```python
from build123d import *

# Parameters (mm, degrees)
SKETCH_1_W           = 55
SKETCH_1_H           = 53
EXTRUDE_1_DEPTH      = 16
SKETCH_3_R           = 2.65
CUT_EXTRUDE_2_DEPTH  = 79.038452061
SKETCH_4_W           = 9.5
SKETCH_4_H           = 12.75
CUT_EXTRUDE_3_DEPTH  = 79.038452061
SKETCH_2_W           = 12
SKETCH_2_H           = 53
CUT_EXTRUDE_4_DEPTH  = 4
SKETCH_5_W           = 12
SKETCH_5_H           = 46
CUT_EXTRUDE_5_DEPTH  = 9
FILLET_1_R           = 2
CUT_EXTRUDE_6_DEPTH  = 79.038452061
FILLET_2_R           = 2
SKETCH_12_W          = 55.94515333
SKETCH_12_H          = 33.208956196
CUT_EXTRUDE_10_DEPTH = 6
SKETCH_13_R          = 1.15
CUT_EXTRUDE_11_DEPTH = 70.756720106
SKETCH_11_W          = 3
SKETCH_11_H          = 46
CUT_EXTRUDE_9_DEPTH  = 13
CUT_EXTRUDE_12_DEPTH = 1
SKETCH_15_R          = 3
SKETCH_15_R_2        = 2.95
CUT_EXTRUDE_13_DEPTH = 12.75
SKETCH_16_R          = 4
CUT_EXTRUDE_14_DEPTH = 2


with BuildPart() as part:
    # 草图1 → 凸台-拉伸1 (new body)
    with BuildSketch(Plane.XY):
        with Locations((-27.5, 26.5)):
            Rectangle(SKETCH_1_W, SKETCH_1_H)
    extrude(amount=EXTRUDE_1_DEPTH)

    # 草图3 → 切除-拉伸2 (cut, through all)
    with BuildSketch(Plane.XZ):
        with Locations(Location((-43, 8, 0), (0, 0, 270))):
            Circle(SKETCH_3_R)
        with Locations(Location((-7, 8, 0), (0, 0, 270))):
            Circle(SKETCH_3_R)
    extrude(amount=-CUT_EXTRUDE_2_DEPTH, mode=Mode.SUBTRACT)

    # 草图4 → 切除-拉伸3 (cut, through all)
    with BuildSketch(Plane.XZ):
        with Locations((-25, 6.375)):
            Rectangle(SKETCH_4_W, SKETCH_4_H)
    extrude(amount=-CUT_EXTRUDE_3_DEPTH, mode=Mode.SUBTRACT)

    # 草图2 → 切除-拉伸4 (cut)
    with BuildSketch(Plane.XY.offset(16)):
        with Locations((-43, 26.5)):
            Rectangle(SKETCH_2_W, SKETCH_2_H)
        with Locations((-6, 26.5)):
            Rectangle(SKETCH_2_W, SKETCH_2_H)
    extrude(amount=-CUT_EXTRUDE_4_DEPTH, mode=Mode.SUBTRACT)

    # 草图5 → 切除-拉伸5 (cut)
    with BuildSketch(Plane.XY.offset(12)):
        with Locations((-43, 30)):
            Rectangle(SKETCH_5_W, SKETCH_5_H)
        with Locations((-6, 30)):
            Rectangle(SKETCH_5_W, SKETCH_5_H)
    extrude(amount=-CUT_EXTRUDE_5_DEPTH, mode=Mode.SUBTRACT)

    # 圆角1
    fillet_1_edges = [part.edges().sort_by_distance(p)[0] for p in [
        (0, 0, 6),
        (0, 53, 1.5),
        (-55, 53, 8),
        (-55, 0, 8),
    ]]
    fillet(fillet_1_edges, radius=FILLET_1_R)

    # 草图6 → 切除-拉伸6 (cut, through all)
    with BuildSketch(Plane.XY.offset(16)):
        with BuildLine():
            Line((-49, 0), (-49, 53))
            Line((-49, 53), (-53, 53))
            ThreePointArc((-53, 53), (-54.414213562, 52.414213562), (-55, 51))
            Line((-55, 51), (-55, 2))
            ThreePointArc((-55, 2), (-54.414213562, 0.585786438), (-53, 0))
            Line((-53, 0), (-49, 0))
        make_face()
    extrude(amount=-CUT_EXTRUDE_6_DEPTH, mode=Mode.SUBTRACT)

    # 圆角2
    fillet_2_edges = [part.edges().sort_by_distance(p)[0] for p in [
        (-49, 53, 1.5),
        (-49, 0, 6),
    ]]
    fillet(fillet_2_edges, radius=FILLET_2_R)

    # 草图12 → 切除-拉伸10 (cut)
    with BuildSketch(Plane(origin=(0, 53, 0), x_dir=(1, 0, 0), z_dir=(0, 1, 0))):
        with Locations((-25.829443508, -5.558164986)):
            Rectangle(SKETCH_12_W, SKETCH_12_H)
    extrude(amount=-CUT_EXTRUDE_10_DEPTH, mode=Mode.SUBTRACT)

    # 草图13 → 切除-拉伸11 (cut, through all)
    with BuildSketch(Plane.XY.offset(16)):
        with Locations((-26.5, 43)):
            Circle(SKETCH_13_R)
        with Locations((-20, 43)):
            Circle(SKETCH_13_R)
    extrude(amount=-CUT_EXTRUDE_11_DEPTH, mode=Mode.SUBTRACT)

    # 草图11 → 切除-拉伸9 (cut)
    with BuildSketch(Plane.XY.offset(16)):
        with Locations((-35.5, 30)):
            Rectangle(SKETCH_11_W, SKETCH_11_H)
        with Locations((-13.5, 30)):
            Rectangle(SKETCH_11_W, SKETCH_11_H)
    extrude(amount=-CUT_EXTRUDE_9_DEPTH, mode=Mode.SUBTRACT)

    # 草图14 → 切除-拉伸12 (cut)
    with BuildSketch(Plane.XY.offset(16)):
        Polygon((-34, 47), (-34, 7), (-37, 7), (-37, 0), (-12, 0), (-12, 7), (-15, 7), (-15, 47), align=None)
    extrude(amount=-CUT_EXTRUDE_12_DEPTH, mode=Mode.SUBTRACT)

    # 草图15 → 切除-拉伸13 (cut)
    with BuildSketch(Plane(origin=(0, 0, 0), x_dir=(-1, 0, 0), z_dir=(0, 0, -1))):
        with Locations((26.5, 43)):
            Circle(SKETCH_15_R)
        with Locations((20, 43)):
            Circle(SKETCH_15_R_2)
    extrude(amount=-CUT_EXTRUDE_13_DEPTH, mode=Mode.SUBTRACT)

    # 草图16 → 切除-拉伸14 (cut)
    with BuildSketch(Plane(origin=(0, 47, 0), x_dir=(1, 0, 0), z_dir=(0, 1, 0))):
        with Locations((-17, -8)):
            Circle(SKETCH_16_R)
        with Locations((-33, -8)):
            Circle(SKETCH_16_R)
    extrude(amount=-CUT_EXTRUDE_14_DEPTH, mode=Mode.SUBTRACT)


solid = part.part
```
Geometry: final body of the model. Coordinates: model frame, mm. A direction names the side the tool comes from. Coordinates: 2 decimals unless noted, no trailing zeros. Order: outer loops, then holes, each group sorted by start corner. A loop starts at its lowest first (then second) coordinate and runs counter-clockwise, first axis right, second up.
Item 1: Section query D-D (x = -33). Output: boundary loops of the cut face in (y, z).
Answer:
outline: (0, 0) - (47, 0) - (47, 4) - (45, 4) - (45, 12) - (47, 12) - (47, 15) - (0, 15) - close
Item 2: Contact query for flat-ended pins moving along their axis: P1, Ø2.5, axis at y = 4.5, z = 13.5, coming from the +X side; P2, Ø3.5, axis at x = -26.5, y = 43, coming from the -Z side; P3, Ø5.5, axis at x = -42, y = 2.5, coming from the +Z side. Output: stop coordinate, or through.
Answer:
P1: stops at x = -12
P2: stops at z = 12.75
P3: stops at z = 12
Item 3: Section query B-B (x = -7). Output: boundary loops of the cut face in (y, z), then the cut area to 3 significant figures.
Answer:
outline: (0, 0) - (47, 0) - (47, 3) - (7, 3) - (7, 5.35) - (0, 5.35) - close; (0, 10.65) - (7, 10.65) - (7, 12) - (0, 12) - close
area: 167 mm2
Item 4: Section query C-C (z = 8). Output: boundary loops of the cut face in (x, y), then the cut area to 3 significant figures.
Answer:
outline: (-49, 2) arc R2 ccw to (-47, 0) - (-45.65, 0) - (-45.65, 7) - (-49, 7) - close; (-40.35, 0) - (-29.75, 0) - (-29.75, 45) - (-34, 45) - (-34, 7) - (-40.35, 7) - close; (-20.25, 0) - (-9.65, 0) - (-9.65, 7) - (-15, 7) - (-15, 45) - (-17.83, 45) arc R2.95 cw to (-20.25, 40.06) - close; (-4.35, 0) - (-2, 0) arc R2 ccw to (0, 2) - (0, 7) - (-4.35, 7) - close
area: 548 mm2
Item 5: Access query for faces 4 (the face through (-43, 4, 12)), 5 (the face through (-20.25, 46.5, 2.8)), 6 (the face through (-6, 4, 12)), 7 (the face through (-8, 27, 3)), 8 (the face through (-17, 46, 12)). Directions: +Z, -Z, +X, -X, +Y, -Y. A direction counts if a zero-diameter tool reaches every point of the face in a straight line with its end or side. Return the directions, or none.
Answer:
face 4: +Z, -X, +Y, -Y
face 5: -Z, +Y, -Y
face 6: +Z, +X, +Y, -Y
face 7: +Z, +X, +Y
face 8: +Y
Item 6: Material intervals for line 1 along X through (y, z) = (4, 8); line 2 along X through (y, z) = (28.5, 9); line 3 along X through (y, z) = (43, 9.5), sorted ascending.
Answer:
line 1: x = -49 to -45.65, -40.35 to -29.75, -20.25 to -9.65, -4.35 to 0
line 2: x = -34 to -29.75, -20.25 to -15
line 3: x = -34 to -29.75, -17.05 to -15
Item 7: Section query A-A (y = 43). Output: boundary loops of the cut face in (x, z).
Answer:
outline: (-49, 0) - (-29.75, 0) - (-29.75, 12.75) - (-27.65, 12.75) - (-27.65, 15) - (-34, 15) - (-34, 3) - (-49, 3) - close; (-25.35, 12.75) - (-21.15, 12.75) - (-21.15, 15) - (-25.35, 15) - close; (-18.85, 12.75) - (-17.05, 12.75) - (-17.05, 0) - (0, 0) - (0, 3) - (-15, 3) - (-15, 15) - (-18.85, 15) - close
Item 8: Draft query along Y for faces 1 (the face through (-9, 7, 6)), 2 (the face through (-30, 0, 7)), 3 (the face through (-17.224, 42.003, 6.286)). Return one class per face: released by +Y, released by -Y, zero draft, split by the parting line, or undercut.
Answer:
face 1: released by +Y
face 2: released by -Y
face 3: undercut
